Geometry check sheet. Reference: the model listing, model coordinates, mm. Face numbers are marked on the shaded views. A direction names the side the tool comes from. Give positions to 0.01 mm unless a question says otherwise; leave off trailing zeros. Write each loop counter-clockwise with the first axis right and the second up, starting at its lowest first coordinate (ties: lowest second). Pieces come first, ordered by that corner, then holes.
(1) Mould release check, pull along X, two halves, no side actions. Record for the marked faces 1, 2 and 3: +X half, -X half, draft (parallel to the pull), parting line (faces both ways), or undercut.
(2) Thickness scan on line 1 along Z through (x, y) = (-12.5, -6.75); line 2 along Z through (x, y) = (33, -10.25); line 3 along Z through (x, y) = (16, -8.5). Record the ranges inside material, lowest first.
(3) Cross-section at C-C (x = -23). Record the boundary of the cut face in (y, z).
(4) Depth check by flat-ended pin: P1, Ø10, axis at x = -2, z = -14.5, coming from the +Y side. Enter the tip coordinate at first touch or a pass-through.
(5) Cross-section at A-A (z = 36). Record the boundary of the cut face in (x, y).
(6) Tool access check on the marked faces 4 and 5. Record the directions out of +Z, -Z, +X, -X, +Y, -Y that give a thin tool (end or side, any length) a straight path to the whole face; none if there is none.
(7) Cross-section at B-B (x = 35). Record the boundary of the cut face in (y, z).
```python
from build123d import *

# Parameters (mm, degrees)
F1_DEPTH = 12.7
F3_D     = 6.35


with BuildPart() as f1:
    # F0 (on Front) → F1 (new body)
    with BuildSketch(Plane.XZ):
        Polygon((-44.45, 25.4), (-44.45, -25.4), (44.45, -25.4), (44.45, 25.4), (9.5911053941, 25.4), align=None)
        with BuildLine():
            Line((9.5911053941, 25.4), (44.45, 25.4))
            Line((44.45, 25.4), (44.45, 49.722302705))
            ThreePointArc((44.45, 49.722302705), (23.794397435, 42.1848996722), (9.5911053941, 25.4))
        make_face()
    extrude(amount=F1_DEPTH)

    # F3 (through all)
    with Locations(Plane(origin=(0, 0, 0), x_dir=(1, 0, 0), z_dir=(0, 1, 0))):
        with Locations((34.925, -37.5611312118)):
            Hole(F3_D / 2)


solid = f1.part
```
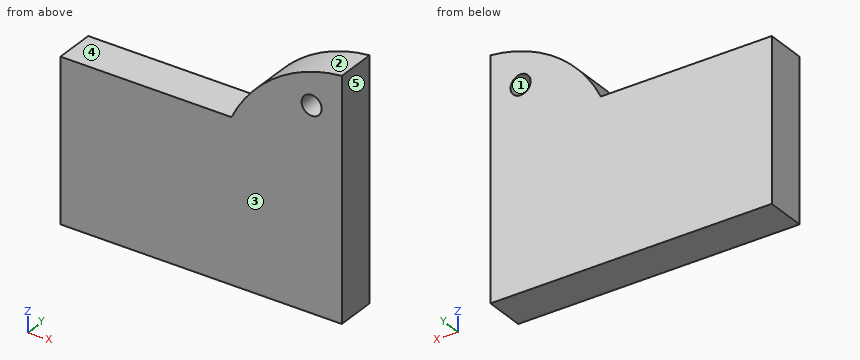
Reply:
1. face 1: undercut
1. face 2: -X half
1. face 3: draft
2. line 1: z = -25.4 to 25.4
2. line 2: z = -25.4 to 35.04, 40.09 to 47.06
2. line 3: z = -25.4 to 35.19
3. outline: (-12.7, -25.4) - (0, -25.4) - (0, 25.4) - (-12.7, 25.4) - close
4. P1: stops at y = 0
5. outline: (16.73, -12.7) - (32.16, -12.7) - (32.16, 0) - (16.73, 0) - close; (37.69, -12.7) - (44.45, -12.7) - (44.45, 0) - (37.69, 0) - close
6. face 4: +Z, -X, +Y, -Y
6. face 5: +Z, -Z, +X, +Y, -Y
7. outline: (-12.7, -25.4) - (0, -25.4) - (0, 34.39) - (-12.7, 34.39) - close; (-12.7, 40.74) - (0, 40.74) - (0, 47.77) - (-12.7, 47.77) - close
